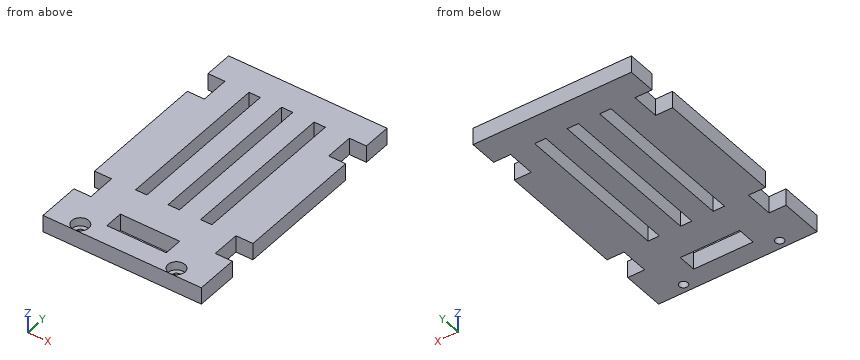
from build123d import *

# Parameters (mm, degrees)
ESQUISSE1_W             = 44
ESQUISSE1_H             = 90
BOSS_EXTRU_1_DEPTH      = 6
ESQUISSE2_W             = 21
ESQUISSE2_H             = 6.5
ESQUISSE2_W_2           = 4
ESQUISSE2_H_2           = 55
ENL_V_MAT_EXTRU_1_DEPTH = 6
ESQUISSE4_W             = 6
ESQUISSE4_H             = 10
ESQUISSE4_H_2           = 45
ESQUISSE4_H_3           = 15
BOSS_EXTRU_2_DEPTH      = 6
ESQUISSE6_R             = 1.5
ENL_V_MAT_EXTRU_3_DEPTH = 6
ESQUISSE8_R             = 2.995
ENL_V_MAT_EXTRU_4_DEPTH = 3


with BuildPart() as part:
    # Esquisse1 → Boss.-Extru.1 (new body)
    with BuildSketch(Plane.XY):
        with Locations((22, 45)):
            Rectangle(ESQUISSE1_W, ESQUISSE1_H)
    extrude(amount=BOSS_EXTRU_1_DEPTH)

    # Esquisse2 → Enlèv. mat.-Extru.1 (cut)
    with BuildSketch(Plane.XY.offset(6)):
        with Locations((22, 10.25)):
            Rectangle(ESQUISSE2_W, ESQUISSE2_H)
        with Locations((22, 52.5)):
            Rectangle(ESQUISSE2_W_2, ESQUISSE2_H_2)
        with Locations((33.5, 52.5)):
            Rectangle(ESQUISSE2_W_2, ESQUISSE2_H_2)
        with Locations((10.5, 52.5)):
            Rectangle(ESQUISSE2_W_2, ESQUISSE2_H_2)
    extrude(amount=-ENL_V_MAT_EXTRU_1_DEPTH, mode=Mode.SUBTRACT)

    # Esquisse4 → Boss.-Extru.2 (add)
    with BuildSketch(Plane.XY.offset(6)):
        with Locations((-3, 85)):
            Rectangle(ESQUISSE4_W, ESQUISSE4_H)
        with Locations((-3, 47.5)):
            Rectangle(ESQUISSE4_W, ESQUISSE4_H_2)
        with Locations((-3, 7.5)):
            Rectangle(ESQUISSE4_W, ESQUISSE4_H_3)
        with Locations((47, 7.5)):
            Rectangle(ESQUISSE4_W, ESQUISSE4_H_3)
        with Locations((47, 47.5)):
            Rectangle(ESQUISSE4_W, ESQUISSE4_H_2)
        with Locations((47, 85)):
            Rectangle(ESQUISSE4_W, ESQUISSE4_H)
    extrude(amount=-BOSS_EXTRU_2_DEPTH)

    # Esquisse6 → Enlèv. mat.-Extru.3 (cut)
    with BuildSketch(Plane.XY.offset(6)):
        with Locations((5, 3)):
            Circle(ESQUISSE6_R)
        with Locations((39, 3)):
            Circle(ESQUISSE6_R)
    extrude(amount=-ENL_V_MAT_EXTRU_3_DEPTH, mode=Mode.SUBTRACT)

    # Esquisse8 → Enlèv. mat.-Extru.4 (cut)
    with BuildSketch(Plane.XY.offset(6)):
        with Locations((5, 3)):
            Circle(ESQUISSE8_R)
        with Locations((39, 3)):
            Circle(ESQUISSE8_R)
    extrude(amount=-ENL_V_MAT_EXTRU_4_DEPTH, mode=Mode.SUBTRACT)


solid = part.part
CAD build for the part. Positions are in the model's coordinates, mm. Round coordinates to 2 decimals unless told otherwise and drop trailing zeros. Write each loop counter-clockwise with the first axis right and the second up, starting at its lowest first coordinate (ties: lowest second). Pieces come first, ordered by that corner, then holes.
(1) Slice it at D-D, the plane y = 3. Write the cut outline in (x, z) (3 decimals), and give its area (3 significant figures).
(2) Slice it at B-B, the plane y = 30. Write the cut outline in (x, z).
(3) Slice it at A-A, the plane x = 27.5. Write the cut outline in (y, z), and give its area (3 significant figures).
(4) Probe line 1 along Y through (x, z) = (-2, 3.55); line 2 along X through (y, z) = (27.5, 1.7); line 3 along X through (y, z) = (72, 2.9). List the from-to ranges inside material, lowest first.
(5) Drop flat-ended pins along their axis: P1, Ø2, axis at y = 74.5, z = 5, coming from the +X side; P2, Ø1.8, axis at x = 5.5, y = 1.5, coming from the +Z side; P3, Ø1.8, axis at y = 22.5, z = 1.5, coming from the -X side; P4, Ø2.5, axis at x = 39, y = 3, coming from the +Z side. Give the stop position or say it passes through.
(6) Slice it at C-C, the plane x = -1.5. Write the cut outline in (y, z).
From the geometry:
1. outline: (-6, 0) - (3.5, 0) - (3.5, 3) - (2.005, 3) - (2.005, 6) - (-6, 6) - close; (6.5, 0) - (37.5, 0) - (37.5, 3) - (36.005, 3) - (36.005, 6) - (7.995, 6) - (7.995, 3) - (6.5, 3) - close; (40.5, 0) - (50, 0) - (50, 6) - (41.995, 6) - (41.995, 3) - (40.5, 3) - close
1. area: 282 mm2
2. outline: (-6, 0) - (8.5, 0) - (8.5, 6) - (-6, 6) - close; (12.5, 0) - (20, 0) - (20, 6) - (12.5, 6) - close; (24, 0) - (31.5, 0) - (31.5, 6) - (24, 6) - close; (35.5, 0) - (50, 0) - (50, 6) - (35.5, 6) - close
3. outline: (0, 0) - (7, 0) - (7, 6) - (0, 6) - close; (13.5, 0) - (90, 0) - (90, 6) - (13.5, 6) - close
3. area: 501 mm2
4. line 1: y = 0 to 15, 25 to 70, 80 to 90
4. line 2: x = -6 to 8.5, 12.5 to 20, 24 to 31.5, 35.5 to 50
4. line 3: x = 0 to 8.5, 12.5 to 20, 24 to 31.5, 35.5 to 44
5. P1: stops at x = 44
5. P2: stops at z = 3
5. P3: stops at x = 0
5. P4: passes through
6. outline: (0, 0) - (15, 0) - (15, 6) - (0, 6) - close; (25, 0) - (70, 0) - (70, 6) - (25, 6) - close; (80, 0) - (90, 0) - (90, 6) - (80, 6) - close
